from build123d import *

# Parameters (mm, degrees)
F0_R     = 25.4
F1_DEPTH = 25.4
F2_R     = 8.779275
F3_DEPTH = 25.4
F4_R     = 5.08
F5_R     = 5.08


with BuildPart() as f1:
    # F0 (on Top) → F1 (new body)
    with BuildSketch(Plane.XY):
        Circle(F0_R)
    extrude(amount=F1_DEPTH)

    # F2 (on face) → F3 (cut)
    with BuildSketch(Plane.XY.offset(25.4)):
        Circle(F2_R)
    extrude(amount=-F3_DEPTH, mode=Mode.SUBTRACT)

    # F4
    f4_edges = [f1.edges().sort_by_distance(p)[0] for p in [
        (-25.4, 0, 25.4),
    ]]
    fillet(f4_edges, radius=F4_R)

    # F5
    f5_edges = [f1.edges().sort_by_distance(p)[0] for p in [
        (-25.4, 0, 0),
    ]]
    fillet(f5_edges, radius=F5_R)


solid = f1.part
Part model, mm, in its own coordinate system. Give positions to 0.01 mm unless a question says otherwise; leave off trailing zeros. Loops run counter-clockwise (first coordinate to the right, second up) from the corner with the lowest first, then second, coordinate; pieces in that order, holes last. Notation, with made-up numbers: M 51,62.5 L 96,62.5 A28 ccw 96,82.5 Z; hole C 70.5,-19 d11. An arc over 180 degrees is marked long. Put each result on its own line as item: value. Start each with the question number.
1) Saw through at C-C (z = 17.5). List the corners of the cut face in (x, y).
2) Probe probe 1 along Y at (x, z) = (0, 11.25); probe 2 along X at (y, z) = (-7.5, 23); probe 3 along X at (y, z) = (-2.5, 12.75). List the from-to ranges inside material, lowest first.
3) Saw through at D-D (z = 3.25). List the corners of the cut face in (x, y), then the cut area to 3 significant figures.
4) Pull direction X, two halves, no side cores. Call faces 1 (the cylindrical face through (-7, -5.3, 12.9)), 2 (the cylindrical face through (-5.506, -24.796, 12.593)), 3 (the flat face through (9, -4, 25.4)): +X half, -X half, draft (parallel to the pull), parting line (faces both ways), or undercut.
5) Saw through at A-A (y = 0). List the corners of the cut face in (x, z).
6) Flat gauge pins, fed straight in: pin 1 (12 mm diameter, centred on x = 7.5, y = -16, fed in from -Z); pin 2 (1.5 mm diameter, centred on x = 15.5, z = 13.5, fed in from +Y); pin 3 (1.5 mm diameter, centred on x = -2.5, z = 14.5, fed in from +Y). Where does each tip first touch, or does it go through?
Numbers:
1. outline: C 0,0 d50.8; hole C 0,0 d17.56
2. probe 1: -25.4 to -8.78, 8.78 to 25.4
2. probe 2: -23.47 to -4.56, 4.56 to 23.47
2. probe 3: -25.28 to -8.42, 8.42 to 25.28
3. outline: C 0,0 d50.12; hole C 0,0 d17.56
3. area: 1,730 mm^2
4. face 1: undercut
4. face 2: parting line
4. face 3: draft
5. outline: M -25.4,5.08 A5.08 ccw -20.32,0 L -8.78,0 L -8.78,25.4 L -20.32,25.4 A5.08 ccw -25.4,20.32 Z; M 8.78,0 L 20.32,0 A5.08 ccw 25.4,5.08 L 25.4,20.32 A5.08 ccw 20.32,25.4 L 8.78,25.4 Z
6. pin 1: z = 0
6. pin 2: y = 20.68
6. pin 3: y = 25.34
